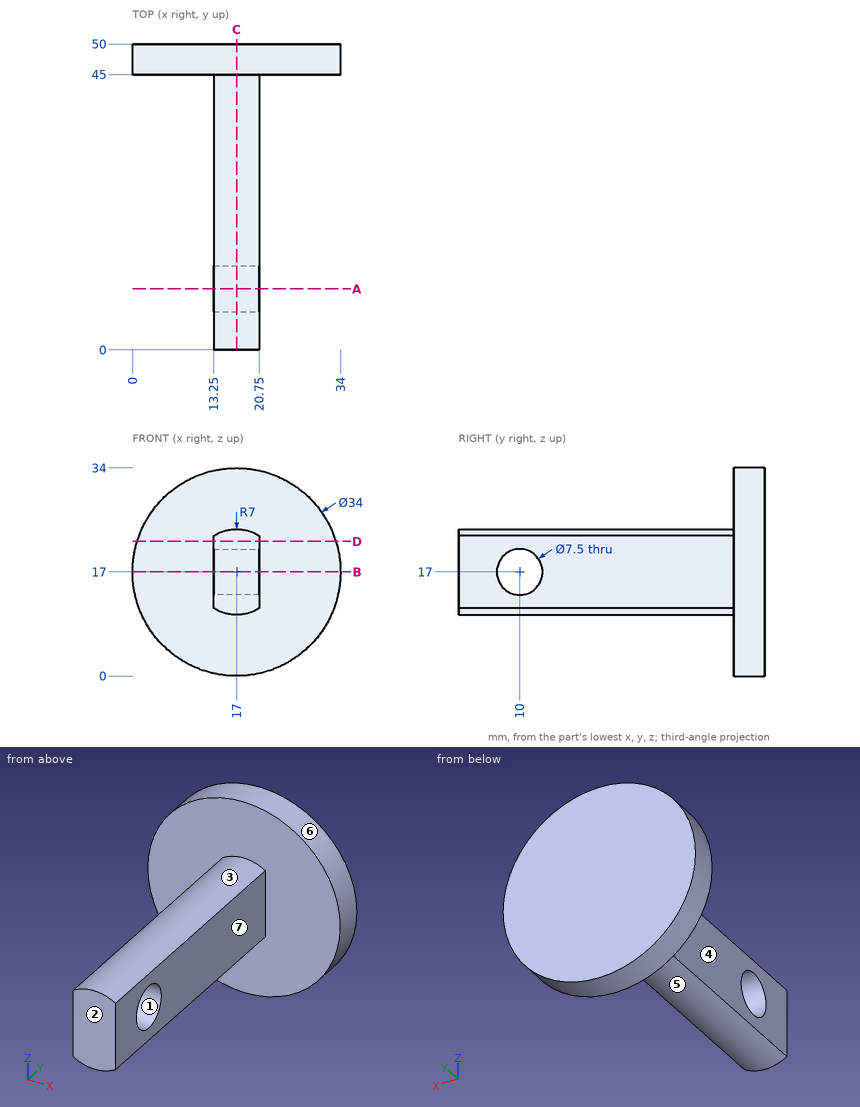
Check sheet for the drawn part. Datum: minimum x, y, z corner. Units: mm. A direction names the side the tool comes from. Round coordinates to 2 decimals unless told otherwise and drop trailing zeros. Order: outer loops, then holes, each group sorted by start corner. A loop starts at its lowest first (then second) coordinate and runs counter-clockwise, first axis right, second up.
(1) Cross-section at C-C, the plane x = 17. Enter the section's corners in (y, z), and give its area (3 significant figures).
(2) Cross-section at D-D, the plane z = 22. Enter the section's corners in (x, y), and give its area (3 significant figures).
(3) Go/stop test with flat-tipped pins: P1, Ø1.5, axis at x = 23.5, z = 5.5, coming from the -Y side; P2, Ø3.5, axis at y = 23.5, z = 19, coming from the -X side; P3, Ø5, axis at x = 20.5, y = 15, coming from the -Z side. Record where each tip stops, or that it passes through.
(4) Cross-section at B-B, the plane z = 17. Enter the section's corners in (x, y).
(5) Cross-section at A-A, the plane y = 10. Enter the section's corners in (x, z), and give its area (3 significant figures).
(6) Access from +Z, -Z, +X, -X, +Y, -Y to the whole of each face (thin tool, end or side, straight path). Record for the marked faces 4, 5, 6 and 7.
(7) Draft check along Z on the marked faces 1, 2 and 3. Enter one of: pulls with the +Z half, pulls with the -Z half, needs draft (parallel to the pull), parting line crosses it, or undercut.
(8) Scan lines: probe 1 along Y at (x, z) = (19.25, 17); probe 2 along Y at (x, z) = (12.5, 19.5); probe 3 along X at (y, z) = (38.5, 17.5). Record each from-to range of solid material in increasing order.
Check sheet entries:
1. outline: (0, 10) - (45, 10) - (45, 0) - (50, 0) - (50, 34) - (45, 34) - (45, 24) - (0, 24) - close; hole circle Ø7.5 at (10, 17)
1. area: 756 mm2
2. outline: (0.75, 45) - (13.25, 45) - (13.25, 0) - (20.75, 0) - (20.75, 45) - (33.25, 45) - (33.25, 50) - (0.75, 50) - close
2. area: 500 mm2
3. P1: stops at y = 45
3. P2: stops at x = 13.25
3. P3: stops at z = 10.07
4. outline: (0, 45) - (13.25, 45) - (13.25, 13.75) - (20.75, 13.75) - (20.75, 45) - (34, 45) - (34, 50) - (0, 50) - close; (13.25, 0) - (20.75, 0) - (20.75, 6.25) - (13.25, 6.25) - close
5. outline: (13.25, 11.09) arc R7 ccw to (20.75, 11.09) - (20.75, 13.25) - (13.25, 13.25) - close; (13.25, 20.75) - (20.75, 20.75) - (20.75, 22.91) arc R7 ccw to (13.25, 22.91) - close
5. area: 43.5 mm2
6. face 4: +Z, -Z, -X, -Y
6. face 5: -Z, -Y
6. face 6: +Y, -Y
6. face 7: +Z, -Z, +X, -Y
7. face 1: undercut
7. face 2: needs draft
7. face 3: pulls with the +Z half
8. probe 1: y = 0 to 6.25, 13.75 to 50
8. probe 2: y = 45 to 50
8. probe 3: x = 13.25 to 20.75
